Read the model definition and answer for the solid it produces. Units are mm, in the model's axes. A direction names the side the tool comes from. Give positions to 0.01 mm unless a question says otherwise; leave off trailing zeros. Order: outer loops, then holes, each group sorted by start corner. A loop starts at its lowest first (then second) coordinate and runs counter-clockwise, first axis right, second up.
```python
from build123d import *

# Parameters (mm, degrees)
F1_DEPTH      = 12.7
F0_W          = 88.9
F0_H          = 88.9
F2_DEPTH      = 12.7
F2_DEPTH_BACK = 508
F3_W          = 889
F3_H          = 12.7
F3_W_2        = 12.7
F3_H_2        = 431.8
F4_DEPTH      = 101.6
F6_W          = 889
F6_H          = 12.7
F6_W_2        = 12.7
F6_H_2        = 431.8
F7_DEPTH      = 25.4


with BuildPart() as f1:
    # F0 (on Top) → F1 (new body)
    with BuildSketch(Plane.XY):
        Polygon((444.5, 304.8), (-444.5, 304.8), (-444.5, 215.9), (-533.4, 215.9), (-533.4, -215.9), (-444.5, -215.9), (-444.5, -304.8), (444.5, -304.8), (444.5, -215.9), (533.4, -215.9), (533.4, 215.9), (444.5, 215.9), align=None)
    extrude(amount=F1_DEPTH)

    # F0 (on Top) → F2 (join, two sides)
    with BuildSketch(Plane.XY) as f2_sk:
        with Locations((-488.95, 260.35)):
            Rectangle(F0_W, F0_H)
        with Locations((-488.95, -260.35)):
            Rectangle(F0_W, F0_H)
        with Locations((488.95, 260.35)):
            Rectangle(F0_W, F0_H)
        with Locations((488.95, -260.35)):
            Rectangle(F0_W, F0_H)
    extrude(amount=F2_DEPTH)
    extrude(f2_sk.sketch, amount=-F2_DEPTH_BACK)

    # F3 (on face) → F4 (join)
    with BuildSketch(Plane(origin=(0, 0, 0), x_dir=(1, 0, 0), z_dir=(0, 0, -1))):
        with Locations((0, 266.7)):
            Rectangle(F3_W, F3_H)
        with Locations((-495.3, 0)):
            Rectangle(F3_W_2, F3_H_2)
        with Locations((0, -266.7)):
            Rectangle(F3_W, F3_H)
        with Locations((495.3, 0)):
            Rectangle(F3_W_2, F3_H_2)
    extrude(amount=F4_DEPTH)

    # F6 (on offset) → F7 (join)
    with BuildSketch(Plane(origin=(0, 0, -355.6), x_dir=(1, 0, 0), z_dir=(0, 0, -1))):
        with Locations((0, 266.7)):
            Rectangle(F6_W, F6_H)
        with Locations((0, -266.7)):
            Rectangle(F6_W, F6_H)
        with Locations((-495.3, 0)):
            Rectangle(F6_W_2, F6_H_2)
        with Locations((495.3, 0)):
            Rectangle(F6_W_2, F6_H_2)
    extrude(amount=F7_DEPTH)


solid = f1.part
```
1) The part is cut by section D-D on y = -243.5. Determine the outline of the cut face in (x, z).
Final values:
outline: (-533.4, -508) - (-444.5, -508) - (-444.5, 0) - (444.5, 0) - (444.5, -508) - (533.4, -508) - (533.4, 12.7) - (-533.4, 12.7) - close
2) The part is cut by section C-C on x = -287. Determine the outline of the cut face in (y, z).
Final values:
outline: (-304.8, 0) - (-273.05, 0) - (-273.05, -101.6) - (-260.35, -101.6) - (-260.35, 0) - (260.35, 0) - (260.35, -101.6) - (273.05, -101.6) - (273.05, 0) - (304.8, 0) - (304.8, 12.7) - (-304.8, 12.7) - close; (-273.05, -381) - (-260.35, -381) - (-260.35, -355.6) - (-273.05, -355.6) - close; (260.35, -381) - (273.05, -381) - (273.05, -355.6) - (260.35, -355.6) - close
3) The part is cut by section B-B on z = -449.5. Determine the outline of the cut face in (x, y), and give its area (3 significant figures).
Final values:
outline: (-533.4, -304.8) - (-444.5, -304.8) - (-444.5, -215.9) - (-533.4, -215.9) - close; (-533.4, 215.9) - (-444.5, 215.9) - (-444.5, 304.8) - (-533.4, 304.8) - close; (444.5, -304.8) - (533.4, -304.8) - (533.4, -215.9) - (444.5, -215.9) - close; (444.5, 215.9) - (533.4, 215.9) - (533.4, 304.8) - (444.5, 304.8) - close
area: 31,600 mm2
4) Given pin 1 (20.5 mm diameter, centred on y = -39.5, z = -365, fed in from +X); pin 2 (7.5 mm diameter, centred on y = 40, z = -371, fed in from -X); pin 3 (5 mm diameter, centred on x = -379, y = -238, fed in from -Z), each flat-ended and moving along its own axis, determine where each tip first touches the part or whether it passes through.
Final values:
pin 1: stops at x = 501.65
pin 2: stops at x = -501.65
pin 3: stops at z = 0
5) Consider L1, parallel to X at y = 75.5, z = -56; L2, parallel to Z at x = -408, y = 273; L3, parallel to Y at x = -305.5, z = -97. Determine where each line is inside the solid, lowest interval first.
Final values:
L1: x = -501.65 to -488.95, 488.95 to 501.65
L2: z = -381 to -355.6, -101.6 to 12.7
L3: y = -273.05 to -260.35, 260.35 to 273.05
6) A tool of negligible diameter and unlimited length cuts with its end or side. For faces 4 (the face through (501.65, 3, -368)), 5 (the face through (-501.65, 3, -50)), 6 (the face through (-6, 273.05, -368)), from which of +Z, -Z, +X, -X, +Y, -Y can it reach the whole face along a straight path? Write none if from no direction.
Final values:
face 4: -Z, +X
face 5: -Z, -X
face 6: -Z, +Y
7) For a pull along Y with two mould halves and no side action, classify faces 1 (the face through (-2, -304.8, 2)), 2 (the face through (-6, 273.05, -50)), 3 (the face through (-488.95, 3, -50)) as released by +Y, released by -Y, zero draft, split by the parting line, or undercut.
Final values:
face 1: released by -Y
face 2: released by +Y
face 3: undercut
8) The part is cut by section A-A on y = -42. Determine the outline of the cut face in (x, z), and give its area (3 significant figures).
Final values:
outline: (-533.4, 0) - (-501.65, 0) - (-501.65, -101.6) - (-488.95, -101.6) - (-488.95, 0) - (488.95, 0) - (488.95, -101.6) - (501.65, -101.6) - (501.65, 0) - (533.4, 0) - (533.4, 12.7) - (-533.4, 12.7) - close; (-501.65, -381) - (-488.95, -381) - (-488.95, -355.6) - (-501.65, -355.6) - close; (488.95, -381) - (501.65, -381) - (501.65, -355.6) - (488.95, -355.6) - close
area: 16,800 mm2
